```python
from build123d import *

# Parameters (mm, degrees)
F0_R     = 21.484759
F0_R_2   = 20.336047
F1_DEPTH = 101.6
F2_R     = 30.47998
F3_DEPTH = 50.8
F4_R     = 12.877415


with BuildPart() as f1:
    # F0 (on Front) → F1 (new body, symmetric)
    with BuildSketch(Plane.XZ):
        Circle(F0_R)
        Circle(F0_R_2, mode=Mode.SUBTRACT)
    extrude(amount=F1_DEPTH, both=True)

    # F2 (on face) → F3 (join)
    with BuildSketch(Plane.XZ.offset(101.6)):
        Circle(F2_R)
    extrude(amount=F3_DEPTH)

    # F4
    f4_edges = [f1.edges().sort_by_distance(p)[0] for p in [
        (-30.47998, -152.4, 0),
    ]]
    fillet(f4_edges, radius=F4_R)


solid = f1.part
```
Source: CAD feature listing. Evaluate the final solid. Frame: model axes, mm. A direction names the side the tool comes from. Coordinates: 2 decimals unless noted, no trailing zeros. Order: outer loops, then holes, each group sorted by start corner. A loop starts at its lowest first (then second) coordinate and runs counter-clockwise, first axis right, second up. Notation, with made-up numbers: (-36.5, -8) - (-13.5, -8) arc R29 cw to (-13.5, 22) - close; hole circle Ø4 at (27, -30). An arc over 180 degrees is marked (long way). One line per item, written item: value.
1) Contact query for flat-ended pins moving along their axis: pin 1 (12 mm diameter, centred on y = -123, z = -12, fed in from -X); pin 2 (3 mm diameter, centred on x = -18, z = -20, fed in from -Y); pin 3 (20.5 mm diameter, centred on x = -0.5, z = 8.5, fed in from +Y); pin 4 (1 mm diameter, centred on y = -11.5, z = -23.5, fed in from -X). Output: stop coordinate, or through.
Computed values:
pin 1: stops at x = -29.88
pin 2: stops at y = -149.77
pin 3: stops at y = -101.6
pin 4: passes through
2) Reachability of faces 1 (the face through (16, 101.6, 13)), 2 (the face through (-4.657, -1.422, -20.974)) from +Z, -Z, +X, -X, +Y, -Y: full face, straight path, thin tool, end or side. Return the list, or none.
Computed values:
face 1: +Z, -Z, +X, -X, +Y
face 2: +Y
3) Cut plane A-A on z = 0. Output: boundary loops of the cut face in (x, y).
Computed values:
outline: (-30.48, -139.52) arc R12.88 ccw to (-17.6, -152.4) - (17.6, -152.4) arc R12.88 ccw to (30.48, -139.52) - (30.48, -101.6) - (21.48, -101.6) - (21.48, 101.6) - (20.34, 101.6) - (20.34, -101.6) - (-20.34, -101.6) - (-20.34, 101.6) - (-21.48, 101.6) - (-21.48, -101.6) - (-30.48, -101.6) - close
4) Cut plane D-D on y = -124.5. Output: boundary loops of the cut face in (x, z).
Computed values:
outline: circle Ø60.96 at (0, 0)
5) Ray query, line 1 (Z direction, x = 0, y = 58); line 2 (X direction, y = -11.5, z = 1); line 3 (Y direction, x = 5.5, z = 10.5). Return the intervals inside material, ascending. Write a range as [from, to].
Computed values:
line 1: z = [-21.48, -20.34], [20.34, 21.48]
line 2: x = [-21.46, -20.31], [20.31, 21.46]
line 3: y = [-152.4, -101.6]
6) Cut plane C-C on x = 0. Output: boundary loops of the cut face in (y, z), plus the area to 3 significant figures.
Computed values:
outline: (-152.4, -17.6) arc R12.88 ccw to (-139.52, -30.48) - (-101.6, -30.48) - (-101.6, -21.48) - (101.6, -21.48) - (101.6, -20.34) - (-101.6, -20.34) - (-101.6, 20.34) - (101.6, 20.34) - (101.6, 21.48) - (-101.6, 21.48) - (-101.6, 30.48) - (-139.52, 30.48) arc R12.88 ccw to (-152.4, 17.6) - close
area: 3,490 mm^2
7) Mould query, pull axis Z, two halves, no side actions, for faces 3 (the face through (-6.607, -120.296, -29.755)), 4 (the face through (0, -101.6, 0)), 5 (the face through (0, -152.4, 0)). Classes: released by +Z, released by -Z, zero draft, split by the parting line, or undercut.
Computed values:
face 3: split by the parting line
face 4: undercut
face 5: zero draft
8) Cut plane B-B on y = -37.5. Output: boundary loops of the cut face in (x, z).
Computed values:
outline: circle Ø42.97 at (0, 0); hole circle Ø40.67 at (0, 0)
